```python
from build123d import *

# Parameters (mm, degrees)
SKETCH_1_R      = 0.4
EXTRUDE_1_DEPTH = 10
SKETCH_2_W      = 80
SKETCH_2_H      = 0.8
EXTRUDE_2_DEPTH = 0.8
FILLET_1_R      = 0.4
SKETCH_3_R      = 0.4
EXTRUDE_3_DEPTH = 3.8
SKETCH_4_R      = 0.4
EXTRUDE_4_DEPTH = 3.8


with BuildPart() as part:
    # 草图1 → 凸台-拉伸1 (new body)
    with BuildSketch(Plane(origin=(0, 0, 0), x_dir=(1, 0, 0), z_dir=(0, 1, 0))):
        with Locations(Location((0, 0, 0), (0, 0, 270))):
            Circle(SKETCH_1_R)
    extrude(amount=EXTRUDE_1_DEPTH)

    # 草图2 → 凸台-拉伸2 (add)
    with BuildSketch(Plane(origin=(0, 10, 0), x_dir=(1, 0, 0), z_dir=(0, 1, 0))):
        Rectangle(SKETCH_2_W, SKETCH_2_H)
    extrude(amount=EXTRUDE_2_DEPTH)

    # 圆角1
    fillet_1_edges = [part.edges().sort_by_distance(p)[0] for p in [
        (40, 10, 0),
        (40, 10.8, 0),
        (-40, 10, 0),
        (-40, 10.8, 0),
    ]]
    fillet(fillet_1_edges, radius=FILLET_1_R - 0.0001)  # a hair under: the kernel refuses the full size

    # 草图3 → 凸台-拉伸3 (add)
    with BuildSketch(Plane.XY.offset(0.4)):
        with Locations((39.6, 10.4)):
            Circle(SKETCH_3_R)
    extrude(amount=EXTRUDE_3_DEPTH)

    # 草图4 → 凸台-拉伸4 (add)
    with BuildSketch(Plane(origin=(0, 0, -0.4), x_dir=(-1, 0, 0), z_dir=(0, 0, -1))):
        with Locations((39.6, 10.4)):
            Circle(SKETCH_4_R)
    extrude(amount=EXTRUDE_4_DEPTH)

    # 草图5 → 旋转1 (revolve)
    with BuildSketch(Plane(origin=(0, 10.4, 0), x_dir=(1, 0, 0), z_dir=(0, 1, 0))):
        Polygon((39.6, -4.2), (39.6, -5.4), (40, -4.2), align=None)
    revolve(axis=Axis((39.6, 10.4, 4.2), (0, 0, 1)))

    # 草图6 → 旋转2 (revolve)
    with BuildSketch(Plane(origin=(0, 10.4, 0), x_dir=(1, 0, 0), z_dir=(0, 1, 0))):
        Polygon((-39.6, 4.2), (-39.6, 5.4), (-40, 4.2), align=None)
    revolve(axis=Axis((-39.6, 10.4, -4.2), (0, 0, -1)))


solid = part.part
```
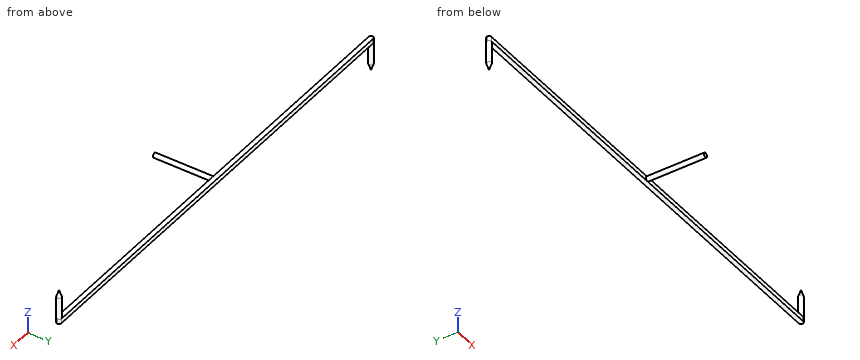
For this review, take the finished solid that the model builds, in its own axes (mm). Round coordinates to 2 decimals unless told otherwise and drop trailing zeros. Write each loop counter-clockwise with the first axis right and the second up, starting at its lowest first coordinate (ties: lowest second). Pieces come first, ordered by that corner, then holes. Notation, with made-up numbers: M 84,-19 L 138,-19 A33 ccw 138,18 Z; hole C 74.25,-11.75 d2. An arc over 180 degrees is marked long. One line per item, written item: value. Start each with the question number.
(1) Insertion check: pin 1 (0.9 mm diameter, centred on x = -19, z = 0, fed in from -Y); pin 2 (5 mm diameter, centred on y = 1.5, z = 0, fed in from -X). Each pin has a flat end and moves straight along its axis. Give the tip position at first contact, or say it passes through.
(2) We need section B-B (x = 9). Give the boundary of the cut face in (y, z).
(3) We need section C-C (y = 2.5). Give the boundary of the cut face in (x, z), and give its area (3 significant figures).
(4) We need section A-A (z = -3.5). Give the boundary of the cut face in (x, y).
(5) Wall thickness on line 1 (Y direction, x = 30, z = 0); line 2 (X direction, y = 1.5, z = 0); line 3 (X direction, y = 5.25, z = -0.25): over which ranges is each line inside the solid? List them lowest first.
Result:
1. pin 1: y = 10
1. pin 2: x = -0.4
2. outline: M 10,-0.4 L 10.8,-0.4 L 10.8,0.4 L 10,0.4 Z
3. outline: C 0,0 d0.8
3. area: 0.503 mm²
4. outline: C -39.6,10.4 d0.8
5. line 1: 10 to 10.8
5. line 2: -0.4 to 0.4
5. line 3: -0.31 to 0.31
